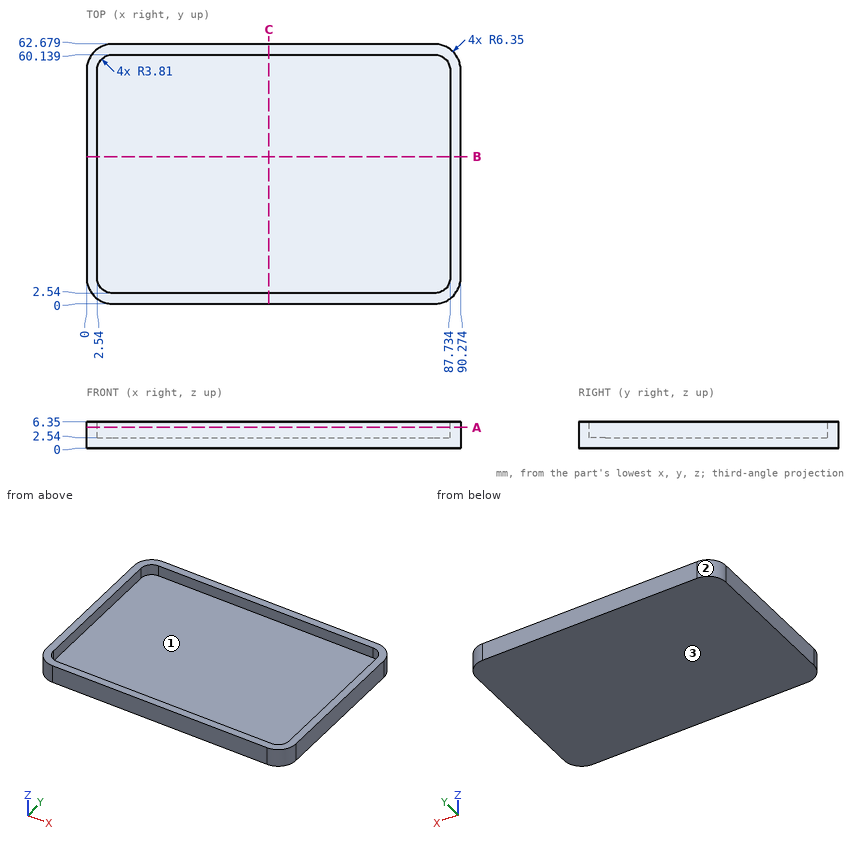
Input: dimensioned drawing with shaded views. Units: mm. Origin: part minimum x, y, z. Coordinates: 2 decimals unless noted, no trailing zeros. Order: outer loops, then holes, each group sorted by start corner. A loop starts at its lowest first (then second) coordinate and runs counter-clockwise, first axis right, second up. Notation, with made-up numbers: (34, -29) -> (59, -29) arc R29 ccw to (59, 9) -> close; hole circle Ø7 at (10.5, -33.75). An arc over 180 degrees is marked (long way). Use CSV: the item, a comma, the result in double quotes.
1) Section B-B on y = 35.5. Output: boundary loops of the cut face in (x, z).
Findings:
outline,"(0, 0) -> (90.27, 0) -> (90.27, 6.35) -> (87.73, 6.35) -> (87.73, 2.54) -> (2.54, 2.54) -> (2.54, 6.35) -> (0, 6.35) -> close"
2) Section C-C on x = 44. Output: boundary loops of the cut face in (y, z), then the cut area to 3 significant figures.
Findings:
outline,"(0, 0) -> (62.68, 0) -> (62.68, 6.35) -> (60.14, 6.35) -> (60.14, 2.54) -> (2.54, 2.54) -> (2.54, 6.35) -> (0, 6.35) -> close"
area,"179 mm^2"
3) Pin query (flat end, axial travel): pin 1 Ø1 at (x, y) = (73.5, 33) entering from +Z. Return the tip coordinate at first contact, or that it passes through.
Findings:
pin 1,"stops at z = 2.54"
4) Mould query, pull axis Y, two halves, no side actions, for the marked faces 1, 2 and 3. Classes: +Y half, -Y half, draft (parallel to the pull), parting line (faces both ways), or undercut.
Findings:
face 1,"undercut"
face 2,"+Y half"
face 3,"draft"
5) Section A-A on z = 5. Output: boundary loops of the cut face in (x, y), then the cut area to 3 significant figures.
Findings:
outline,"(0, 6.35) arc R6.35 ccw to (6.35, 0) -> (83.92, 0) arc R6.35 ccw to (90.27, 6.35) -> (90.27, 56.33) arc R6.35 ccw to (83.92, 62.68) -> (6.35, 62.68) arc R6.35 ccw to (0, 56.33) -> close; hole (2.54, 6.35) arc R3.81 ccw to (6.35, 2.54) -> (83.92, 2.54) arc R3.81 ccw to (87.73, 6.35) -> (87.73, 56.33) arc R3.81 ccw to (83.92, 60.14) -> (6.35, 60.14) arc R3.81 ccw to (2.54, 56.33) -> close"
area,"729 mm^2"
6) Line query: line 1 (Y direction, x = 23, z = 3.5); line 2 (X direction, y = 30.5, z = 3.75); line 3 (Z direction, x = 46.5, y = 54.5). Output: solid intervals per line, ascending.
Findings:
line 1,"y = 0 to 2.54, 60.14 to 62.68"
line 2,"x = 0 to 2.54, 87.73 to 90.27"
line 3,"z = 0 to 2.54"
